Build history of the part. All positions in model axes, mm. Face numbers are marked on the shaded views. A direction names the side the tool comes from. Round coordinates to 2 decimals unless told otherwise and drop trailing zeros. Loops run counter-clockwise (first coordinate to the right, second up) from the corner with the lowest first, then second, coordinate; pieces in that order, holes last. Notation, with made-up numbers: (46.25, -7.75) - (92.25, -7.75) arc R33 cw to (92.25, 28.25) - close; hole circle Ø6 at (11.25, -1). An arc over 180 degrees is marked (long way). Put each result on its own line as item: value. Start each with the question number.
from build123d import *

# Parameters (mm, degrees)
F1_DEPTH      = 34.29
F1_DEPTH_BACK = 10.16
F3_DEPTH      = 27.94
F3_DEPTH_BACK = 3.81
F4_R          = 12.446
F5_DEPTH      = 39.37
F6_W          = 52.9463477433
F6_H          = 63.3781589568
F7_DEPTH      = 25.4
F9_DEPTH      = 24.13
F11_DEPTH     = 50.8
F12_W         = 7.2337351131
F12_H         = 31.75
F13_DEPTH     = 25.4


with BuildPart() as f1:
    # F0 (on Front) → F1 (new body, two sides)
    with BuildSketch(Plane.XZ) as f1_sk:
        Polygon((-19.05, 5.08), (-19.05, 0), (0, 0), (0, -35.052), (64.77, -35.052), (0, 5.08), align=None)
    extrude(amount=F1_DEPTH)
    extrude(f1_sk.sketch, amount=-F1_DEPTH_BACK)

    # F2 (on Front) → F3 (join, two sides)
    with BuildSketch(Plane.XZ) as f3_sk:
        Polygon((-13.97, 51.8359215686), (-13.97, 13.7359215686), (64.77, -35.052), (126.2605063291, -35.052), align=None)
    extrude(amount=F3_DEPTH)
    extrude(f3_sk.sketch, amount=-F3_DEPTH_BACK)

    # F4 (on face) → F5 (cut)
    with BuildSketch(Plane(origin=(0, 0, 0), x_dir=(1, 0, 0), z_dir=(0, 0, -1))):
        with Locations((-12.446, 12.065)):
            Circle(F4_R)
    extrude(amount=-F5_DEPTH, mode=Mode.SUBTRACT)

    # F6 (on face) → F7 (cut)
    with BuildSketch(Plane(origin=(0, 0, 39.37), x_dir=(1, 0, 0), z_dir=(0, 0, -1))):
        with Locations((-10.5953570455, 10.2349836379)):
            Rectangle(F6_W, F6_H)
    extrude(amount=-F7_DEPTH, mode=Mode.SUBTRACT)

    # F8 (on Front) → F9 (cut)
    with BuildSketch(Plane.XZ):
        Polygon((154.4132999091, -56.9777707196), (-10.16, 44.993136675), (-10.16, 11.3752156863), (100.156528693, -56.9777707196), align=None)
    extrude(amount=F9_DEPTH, mode=Mode.SUBTRACT)

    # F10 (on face) → F11 (cut)
    with BuildSketch(Plane.XZ.offset(34.29)):
        Polygon((0, -3.81), (0, -35.052), (56.7722151899, -35.052), (6.35, -3.81), align=None)
    extrude(amount=-F11_DEPTH, mode=Mode.SUBTRACT)

    # F12 (on face) → F13 (cut)
    with BuildSketch(Plane(origin=(0, 0, -35.052), x_dir=(1, 0, 0), z_dir=(0, 0, -1))):
        with Locations((122.6436387726, 12.065)):
            Rectangle(F12_W, F12_H)
    extrude(amount=-F13_DEPTH, mode=Mode.SUBTRACT)


solid = f1.part
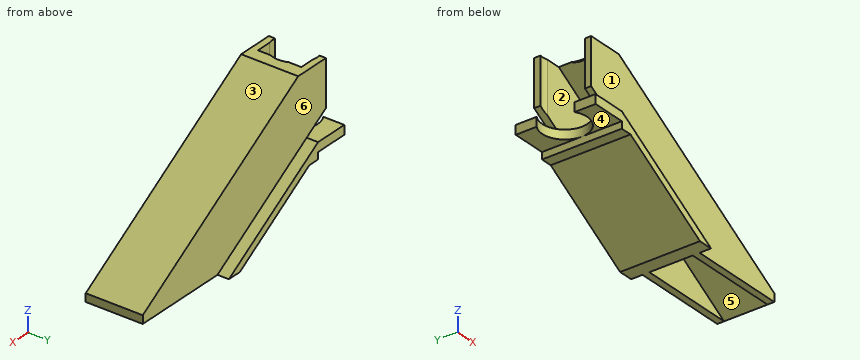
1) Slice it at D-D, the plane y = -9.5. Write the cut outline in (x, z), and give its area (3 significant figures).
2) Which spindle directions (+Z, -Z, +X, -X, +Y, -Y) get a long thin tool onto all of the face, cutting with end or side? Do the marked faces 4, 5 and 6. Say none if no direction does.
3) Slice it at A-A, the plane z = -14. Write the cut outline in (x, y), and give its area (3 significant figures).
4) Slice it at B-B, the plane x = 4. Write the cut outline in (y, z), and give its area (3 significant figures).
5) Slice it at C-C, the plane y = 6. Write the cut outline in (x, z), and give its area (3 significant figures).
6) Pull direction Y, two halves, no side cores. Call the marked faces 1, 2 and 3: pulls with the +Y half, pulls with the -Y half, needs draft (parallel to the pull), parting line crosses it, or undercut.
7) Drop flat-ended pins along their axis: pin 1 Ø2 at (x, y) = (78, -27.5) entering from +Z; pin 2 Ø4 at (x, y) = (27.5, -3.5) entering from -Z; pin 3 Ø3 at (y, z) = (-27, 27) entering from -X. Give the stop position or say it passes through.
8) Drill centre lines: line 1 (Y direction, x = 6, z = 24.5); line 2 (Z direction, x = 42, y = -7); line 3 (Z direction, x = 61.5, y = -6.5). Where is each one in solid material? Low to high. Write a range as [from, to].
Taken from the geometry:
1. outline: (-0.27, 0) - (0, 0) - (0, -3.81) - (6.35, -3.81) - (56.77, -35.05) - (64.77, -35.05) - (0, 5.08) - (-0.27, 5.08) - close; (-0.27, 38.86) - (119.03, -35.05) - (119.03, -30.57) - (6.15, 39.37) - (-0.27, 39.37) - close
1. area: 837 mm2
2. face 4: -Z, -X, +Y, -Y
2. face 5: none
2. face 6: +Z, +X, +Y
3. outline: (22.8, -34.29) - (30.79, -34.29) - (30.79, -27.94) - (92.28, -27.94) - (92.28, 3.81) - (30.79, 3.81) - (30.79, 10.16) - (22.8, 10.16) - close; hole (30.79, -24.13) - (85.05, -24.13) - (85.05, 0) - (30.79, 0) - close
3. area: 999 mm2
4. outline: (-34.29, -3.81) - (10.16, -3.81) - (10.16, 2.6) - (3.81, 2.6) - (3.81, 39.37) - (-27.94, 39.37) - (-27.94, 2.6) - (-34.29, 2.6) - close; hole (-24.13, 2.6) - (0, 2.6) - (0, 36.22) - (-24.13, 36.22) - close
4. area: 641 mm2
5. outline: (-19.05, 0) - (0, 0) - (0, -3.81) - (6.35, -3.81) - (56.77, -35.05) - (64.77, -35.05) - (0, 5.08) - (-19.05, 5.08) - close
5. area: 410 mm2
6. face 1: pulls with the -Y half
6. face 2: undercut
6. face 3: needs draft
7. pin 1: stops at z = -4.53
7. pin 2: stops at z = -18.15
7. pin 3: stops at x = -13.97
8. line 1: y = [-27.94, -24.13], [0, 3.81]
8. line 2: z = [-25.9, -20.94], [12.67, 17.16]
8. line 3: z = [-35.05, -33.03], [0.59, 5.07]
